For this review, take the finished solid that the model builds, in its own axes (mm). Coordinates: 2 decimals unless noted, no trailing zeros. Loops run counter-clockwise (first coordinate to the right, second up) from the corner with the lowest first, then second, coordinate; pieces in that order, holes last. Notation, with made-up numbers: (32.25, 52.5) -> (61.25, 52.5) arc R31 ccw to (61.25, 78.5) -> close; hole circle Ø4 at (21, 33.5). An arc over 180 degrees is marked (long way). Use a Markdown table: item, result.
from build123d import *

# Parameters (mm, degrees)
F0_W     = 25
F0_H     = 25
F1_DEPTH = 2
F3_DEPTH = 2


with BuildPart() as f1:
    # F0 (on Front) → F1 (new body)
    with BuildSketch(Plane.XZ):
        Rectangle(F0_W, F0_H)
    extrude(amount=F1_DEPTH)

    # F2 (on Right) → F3 (join)
    with BuildSketch(Plane.YZ):
        Polygon((-10, 12.2555047274), (0, 12.2555047274), (50, 12.2555047274), (50, 62.2555047274), (-10, 62.2555047274), align=None)
    extrude(amount=F3_DEPTH)


solid = f1.part
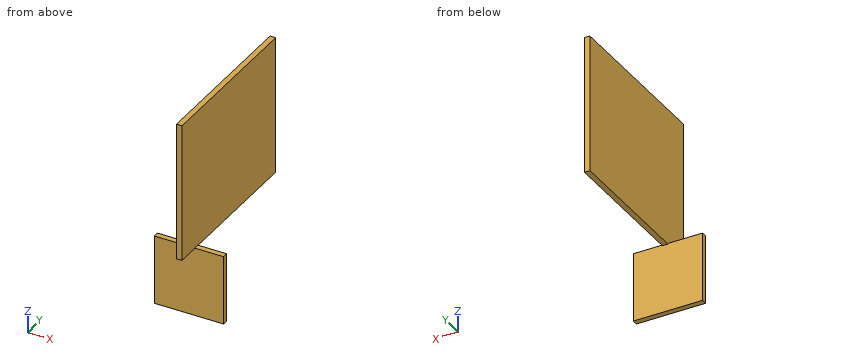
(1) Take a section at B-B on x = 8.5. Write out the cut boundary in (y, z).
Found:
| item | result |
|---|---|
| outline | (-2, -12.5) -> (0, -12.5) -> (0, 12.5) -> (-2, 12.5) -> close |
(2) For line 1 along X through (y, z) = (5, 24); line 2 along Y through (x, z) = (3.5, 4), list the stretches that pass through material, from the lowest coordinate up.
Found:
| item | result |
|---|---|
| line 1 | x = 0 to 2 |
| line 2 | y = -2 to 0 |
(3) For pin 1 Ø6 at (y, z) = (22, 19.5) entering from -X; pin 2 Ø0.6 at (x, y) = (1, -5) entering from -Z; pin 3 Ø15 at (y, z) = (26, 36.5) entering from +X, all flat-tipped, find the tip position at first contact; note any pin that passes through.
Found:
| item | result |
|---|---|
| pin 1 | stops at x = 0 |
| pin 2 | stops at z = 12.26 |
| pin 3 | stops at x = 2 |
(4) Take a section at A-A on z = 0.5. Write out the cut boundary in (x, y).
Found:
| item | result |
|---|---|
| outline | (-12.5, -2) -> (12.5, -2) -> (12.5, 0) -> (-12.5, 0) -> close |
